from build123d import *

# Parameters (mm, degrees)
F0_W     = 1230
F0_H     = 700
F1_DEPTH = 5
F2_W     = 1230
F2_H     = 300
F3_DEPTH = 40
F4_R     = 40
F5_W     = 20
F5_H     = 500
F6_DEPTH = 25
F7_W     = 570
F7_H     = 20
F8_DEPTH = 25


with BuildPart() as f1:
    # F0 (on Front) → F1 (new body)
    with BuildSketch(Plane.XZ):
        Rectangle(F0_W, F0_H)
    extrude(amount=F1_DEPTH)

    # F2 (on face) → F3 (join)
    with BuildSketch(Plane(origin=(0, 0, 0), x_dir=(-1, 0, 0), z_dir=(0, 1, 0))):
        with Locations((0, -150)):
            Rectangle(F2_W, F2_H)
    extrude(amount=F3_DEPTH)

    # F4
    f4_edges = [f1.edges().sort_by_distance(p)[0] for p in [
        (615, 40, -150),
        (-615, 40, -150),
    ]]
    fillet(f4_edges, radius=F4_R)

    # F5 (on face) → F6 (join)
    with BuildSketch(Plane(origin=(0, 40, 0), x_dir=(-1, 0, 0), z_dir=(0, 1, 0))):
        with Locations((-200, -67.909449)):
            Rectangle(F5_W, F5_H)
        with Locations((200, -67.909449)):
            Rectangle(F5_W, F5_H)
    extrude(amount=F6_DEPTH)

    # F7 (on face) → F8 (join)
    with BuildSketch(Plane(origin=(0, 65, 0), x_dir=(-1, 0, 0), z_dir=(0, 1, 0))):
        with Locations((0, 82.090551)):
            Rectangle(F7_W, F7_H)
        with Locations((0, -217.909449)):
            Rectangle(F7_W, F7_H)
    extrude(amount=F8_DEPTH)


solid = f1.part
CAD build for the part. Positions are in the model's coordinates, mm. A direction names the side the tool comes from. Coordinates: 2 decimals unless noted, no trailing zeros. Write each loop counter-clockwise with the first axis right and the second up, starting at its lowest first coordinate (ties: lowest second). Pieces come first, ordered by that corner, then holes. Notation, with made-up numbers: M 76.5,5 L 80.5,5 A15 ccw 80.5,14 Z; hole C 60,-32.75 d1. An arc over 180 degrees is marked long. Answer as a JSON object with one key per item and string values. Group by question number.
1) Saw through at D-D (x = 333). Write the cut outline in (y, z), plus the area to 3 significant figures.
2) Saw through at B-B (y = 78.5). Write the cut outline in (x, z), plus the area to 3 significant figures.
3) Saw through at A-A (z = 147). Write the cut outline in (x, y), plus the area to 3 significant figures.
4) Saw through at C-C (z = -180.5). Write the cut outline in (x, y), plus the area to 3 significant figures.
5) Tool access for faces 1 (the face through (4, 77, 92.091)), 2 (the face through (4, 77, -227.909)), 3 (the face through (603.594, 27.972, -147.9)), 4 (the face through (4, 77, -207.909)), 5 (the face through (-9, -5, 5)): list every direction of +Z, -Z, +X, -X, +Y, -Y with a clear straight run to the whole face (end or side of a thin tool).
6) Wall check: line 1 (X direction, y = 58.5, z = -259.5); line 2 (Y direction, x = -184, z = 74.5); line 3 (Y direction, x = 14, z = 268). Give the ranges that are in metal, low to high. Write a range as from..to.
7) Pin check, flat tips, straight feed: pin 1 Ø6 at (x, z) = (-203.5, 118.5) entering from +Y; pin 2 Ø20 at (x, y) = (53.5, 76) entering from +Z; pin 3 Ø6 at (x, y) = (-195.5, 53.5) entering from +Z. Stop position of each tip, or through.
Values follow:
{
 "1": {"outline": "M -5,-350 L 0,-350 L 0,-300 L 40,-300 L 40,0 L 0,0 L 0,350 L -5,350 Z", "area": "15,500 mm2"},
 "2": {"outline": "M -285,-227.91 L 285,-227.91 L 285,-207.91 L -285,-207.91 Z; M -285,72.09 L 285,72.09 L 285,92.09 L -285,92.09 Z", "area": "22,800 mm2"},
 "3": {"outline": "M -615,-5 L 615,-5 L 615,0 L -615,0 Z; M -210,40 L -190,40 L -190,65 L -210,65 Z; M 190,40 L 210,40 L 210,65 L 190,65 Z", "area": "7,150 mm2"},
 "4": {"outline": "M -615,-5 L 615,-5 L 615,0 A40 ccw 575,40 L 210,40 L 210,65 L 190,65 L 190,40 L -190,40 L -190,65 L -210,65 L -210,40 L -575,40 A40 ccw -615,0 Z", "area": "55,700 mm2"},
 "5": {"face 1": "+Z, +X, -X, +Y", "face 2": "-Z, +X, -X, +Y", "face 3": "+Z, -Z, +X, +Y", "face 4": "+X, -X, +Y", "face 5": "+Z, -Z, +X, -X, -Y"},
 "6": {"line 1": "x = -210..-190, 190..210", "line 2": "y = -5..0, 65..90", "line 3": "y = -5..0"},
 "7": {"pin 1": "stops at y = 65", "pin 2": "stops at z = 92.09", "pin 3": "stops at z = 182.09"}
}
